from build123d import *

# Parameters (mm, degrees)
SKETCH1_R           = 8.5
SKETCH1_R_2         = 2
BOSS_EXTRUDE1_DEPTH = 2


with BuildPart() as part:
    # Sketch1 → Boss-Extrude1 (new body)
    with BuildSketch(Plane.XY):
        with BuildLine():
            ThreePointArc((-15.03512775, 19.973605922), (-17.88515711, 17.467717514), (-20.323051095, 14.559312971))
            ThreePointArc((-20.323051095, 14.559312971), (-23.11408994, 9.525694004), (-24.68, 3.987179454))
            ThreePointArc((-24.68, 3.987179454), (-29, 0), (-24.68, -3.987179454))
            ThreePointArc((-24.68, -3.987179454), (-17.67766953, -17.67766953), (-3.987179454, -24.68))
            ThreePointArc((-3.987179454, -24.68), (0, -29), (3.987179454, -24.68))
            ThreePointArc((3.987179454, -24.68), (23.000009149, 9.797937495), (-15.03512775, 19.973605922))
        make_face()
        Circle(SKETCH1_R, mode=Mode.SUBTRACT)
        with Locations((0, -25)):
            Circle(SKETCH1_R_2, mode=Mode.SUBTRACT)
        with Locations((15.0260191, 15.0260191)):
            Circle(SKETCH1_R_2, mode=Mode.SUBTRACT)
        with Locations((-25, 0)):
            Circle(SKETCH1_R_2, mode=Mode.SUBTRACT)
    extrude(amount=BOSS_EXTRUDE1_DEPTH)


solid = part.part
For this review, take the finished solid that the model builds, in its own axes (mm). Round coordinates to 2 decimals unless told otherwise and drop trailing zeros. Order: outer loops, then holes, each group sorted by start corner. A loop starts at its lowest first (then second) coordinate and runs counter-clockwise, first axis right, second up. Notation, with made-up numbers: (82.5, 49) -> (130.5, 49) arc R8 cw to (130.5, 59) -> close; hole circle Ø9 at (41, -22.5). An arc over 180 degrees is marked (long way). Put each result on its own line as item: value.
Q1. Add section C-C on z = 1.7. Write out the cut boundary in (x, y).
Check result:
outline: (-24.68, -3.99) arc R25 ccw to (-3.99, -24.68) arc R4 ccw (long way) to (3.99, -24.68) arc R25 ccw (long way) to (-24.68, 3.99) arc R4 ccw (long way) to start; hole circle Ø4 at (-25, 0); hole circle Ø17 at (0, 0); hole circle Ø4 at (0, -25); hole circle Ø4 at (15.03, 15.03)
Q2. Add section D-D on x = -6. Write out the cut boundary in (y, z), plus the area to 3 significant figures.
Check result:
outline: (-24.27, 0) -> (-6.02, 0) -> (-6.02, 2) -> (-24.27, 2) -> close; (6.02, 0) -> (24.27, 0) -> (24.27, 2) -> (6.02, 2) -> close
area: 73.0 mm2
Q3. Insertion check: pin 1 Ø4 at (x, y) = (-1.5, -5) entering from -Z; pin 2 Ø10 at (x, y) = (4.5, 4) entering from -Z; pin 3 Ø1 at (x, z) = (-8.5, 1) entering from +Y; pin 4 Ø1 at (x, z) = (-14, 1) entering from +Y. Each pin has a flat end and moves straight along its axis. Give the tip position at first contact, or say it passes through.
Check result:
pin 1: through
pin 2: z = 0
pin 3: y = 23.69
pin 4: y = 21.04
Q4. Mouldability with a two-part tool opening along X and no side actions: class faces 1 (the cylindrical face through (-27, 0, 1)), 2 (the cylindrical face through (-17.832, -17.522, 0.986)), 3 (the cylindrical face through (0, -29, 1)) as pulls with the +X half, pulls with the -X half, needs draft (parallel to the pull), parting line crosses it, or undercut.
Check result:
face 1: undercut
face 2: pulls with the -X half
face 3: parting line crosses it
Q5. For probe 1 along Y at (x, z) = (0, 0.9); probe 2 along Y at (x, z) = (-25, 0.9); probe 3 along X at (y, z) = (-0.5, 1.85) (1 decimal), list the stretches that pass through material, from the lowest coordinate up. Write a range as [from, to].
Check result:
probe 1: [-29, -27], [-23, -8.5], [8.5, 25]
probe 2: [-4, -2], [2, 4]
probe 3: [-29, -26.9], [-23.1, -8.5], [8.5, 25]
Q6. Add section A-A on y = 0. Write out the cut boundary in (x, z).
Check result:
outline: (-29, 0) -> (-27, 0) -> (-27, 2) -> (-29, 2) -> close; (-23, 0) -> (-8.5, 0) -> (-8.5, 2) -> (-23, 2) -> close; (8.5, 0) -> (25, 0) -> (25, 2) -> (8.5, 2) -> close
